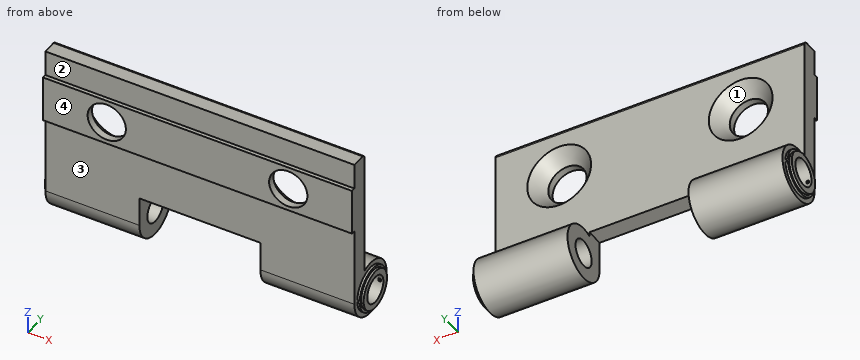
```python
from build123d import *

# Parameters (mm, degrees)
BOSS_EXTRUDE1_DEPTH    = 19.166666667
BOSS_EXTRUDE2_DEPTH    = 0.5
SKETCH3_W              = 5.123475383
SKETCH3_H              = 3.5
BOSS_EXTRUDE3_DEPTH    = 24.666666667
BOSS_EXTRUDE4_START    = 19.166666667
BOSS_EXTRUDE4_DEPTH    = 19.166666667
BOSS_EXTRUDE5_START    = 0.5
BOSS_EXTRUDE5_DEPTH    = 0.5
BOSS_EXTRUDE6_START    = 0.5
BOSS_EXTRUDE6_DEPTH    = 0.5
CUT_EXTRUDE1_DEPTH     = 19.166666667
SKETCH8_W              = 63
SKETCH8_H              = 3.5
BOSS_EXTRUDE7_DEPTH    = 0.338316441
SKETCH9_W              = 63
SKETCH9_H              = 5.461791824
BOSS_EXTRUDE8_DEPTH    = 0.8
CUT_EXTRUDE2_DEPTH     = 5.123475383
SKETCH11_W             = 63
SKETCH11_H             = 4.3
BOSS_EXTRUDE9_DEPTH    = 25.538208176
CUT_EXTRUDE3_DEPTH     = 0.338316441
SKETCH13_W             = 63
SKETCH13_H             = 0.8
CUT_EXTRUDE4_DEPTH     = 10.788208176
SKETCH14_W             = 24.666666666
SKETCH14_H             = 3.5
CUT_EXTRUDE5_DEPTH     = 0.538208176
BOSS_EXTRUDE10_START   = 0.5
SKETCH15_R             = 4
SKETCH15_R_2           = 2.75
BOSS_EXTRUDE10_DEPTH   = 0.5
SKETCH16_R             = 4
BOSS_EXTRUDE11_DEPTH   = 0.5
SKETCH17_W             = 5.25
SKETCH17_H             = 0.8
CUT_EXTRUDE6_DEPTH     = 72.95832127
F_10_CLEARANCE_HOLE1_D = 5.5
HOLE1_AT_2_COUNT       = 2
HOLE1_AT_2_PITCH       = 37
FILLET1_R              = 0.8
SCALE1_SCALE           = 0.3333


with BuildPart() as part:
    # Sketch1 → Boss-Extrude1 (new body)
    with BuildSketch(Plane(origin=(-12.333333333, 0, 0), x_dir=(0, 0, -1), z_dir=(1, 0, 0))):
        with BuildLine():
            Line((-5.123475383, 3.5), (-5.123475383, 0))
            Line((-5.123475383, 0), (0, 0))
            ThreePointArc((0, 0), (3.102418411, 10.041475531), (-5.123475383, 3.5))
        make_face()
    extrude(amount=-BOSS_EXTRUDE1_DEPTH)

    # Sketch2 → Boss-Extrude2 (add)
    with BuildSketch(Plane.ZY.offset(31.5)):
        with BuildLine():
            Line((-0.3, 9.989988864), (-0.3, 8.233587387))
            ThreePointArc((-0.3, 8.233587387), (0, 8.25), (0.3, 8.233587387))
            Line((0.3, 8.233587387), (0.3, 9.989988864))
            ThreePointArc((0.3, 9.989988864), (4.5, 5.5), (0.3, 1.010011136))
            Line((0.3, 1.010011136), (0.3, 2.766412613))
            ThreePointArc((0.3, 2.766412613), (0, 2.75), (-0.3, 2.766412613))
            Line((-0.3, 2.766412613), (-0.3, 1.010011136))
            ThreePointArc((-0.3, 1.010011136), (-4.5, 5.5), (-0.3, 9.989988864))
        make_face()
    extrude(amount=BOSS_EXTRUDE2_DEPTH)

    # Sketch3 → Boss-Extrude3 (add)
    with BuildSketch(Plane(origin=(-12.333333333, 0, 0), x_dir=(0, 0, -1), z_dir=(1, 0, 0))):
        with Locations((-2.561737692, 1.75)):
            Rectangle(SKETCH3_W, SKETCH3_H)
    extrude(amount=BOSS_EXTRUDE3_DEPTH)

    # Sketch4 → Boss-Extrude4 (add)
    with BuildSketch(Plane(origin=(12.333333333, 0, 0), x_dir=(0, 0, -1), z_dir=(1, 0, 0)).offset(BOSS_EXTRUDE4_START)):
        with BuildLine():
            Line((0, 0), (-5.123475383, 0))
            Line((-5.123475383, 0), (-5.123475383, 3.5))
            ThreePointArc((-5.123475383, 3.5), (3.102418411, 10.041475531), (0, 0))
        make_face()
        with BuildLine():
            Line((-1.887458609, 3.5), (0, 3.5))
            Line((0, 3.5), (0, 2.75))
            ThreePointArc((0, 2.75), (1.015504801, 8.055631038), (-1.887458609, 3.5))
        make_face(mode=Mode.SUBTRACT)
    extrude(amount=-BOSS_EXTRUDE4_DEPTH)

    # Sketch5 → Boss-Extrude5 (add)
    with BuildSketch(Plane(origin=(31.5, 0, 0), x_dir=(0, 0, -1), z_dir=(1, 0, 0)).offset(BOSS_EXTRUDE5_START)):
        with BuildLine():
            Line((-0.3, 9.989988864), (-0.3, 8.233587387))
            ThreePointArc((-0.3, 8.233587387), (-2.75, 5.5), (-0.3, 2.766412613))
            Line((-0.3, 2.766412613), (-0.3, 1.010011136))
            ThreePointArc((-0.3, 1.010011136), (-4.5, 5.5), (-0.3, 9.989988864))
        make_face()
    extrude(amount=-BOSS_EXTRUDE5_DEPTH)

    # Sketch6 → Boss-Extrude6 (add)
    with BuildSketch(Plane(origin=(31.5, 0, 0), x_dir=(0, 0, -1), z_dir=(1, 0, 0)).offset(BOSS_EXTRUDE6_START)):
        with BuildLine():
            Line((0.3, 1.010011136), (0.3, 2.766412613))
            ThreePointArc((0.3, 2.766412613), (2.75, 5.5), (0.3, 8.233587387))
            Line((0.3, 8.233587387), (0.3, 9.989988864))
            ThreePointArc((0.3, 9.989988864), (4.5, 5.5), (0.3, 1.010011136))
        make_face()
    extrude(amount=-BOSS_EXTRUDE6_DEPTH)

    # Sketch7 → Cut-Extrude1 (cut)
    with BuildSketch(Plane(origin=(31.5, 0, 0), x_dir=(0, 0, -1), z_dir=(1, 0, 0))):
        with BuildLine():
            Line((0, 3.5), (-1.887458609, 3.5))
            ThreePointArc((-1.887458609, 3.5), (-1.015504801, 2.944368962), (0, 2.75))
            Line((0, 2.75), (0, 3.5))
        make_face()
    extrude(amount=-CUT_EXTRUDE1_DEPTH, mode=Mode.SUBTRACT)

    # Sketch8 → Boss-Extrude7 (add)
    with BuildSketch(Plane.XY.offset(5.123475383)):
        with Locations((0, 1.75)):
            Rectangle(SKETCH8_W, SKETCH8_H)
    extrude(amount=BOSS_EXTRUDE7_DEPTH)

    # Sketch9 → Boss-Extrude8 (add)
    with BuildSketch(Plane.XZ):
        with Locations((0, 2.730895912)):
            Rectangle(SKETCH9_W, SKETCH9_H)
    extrude(amount=BOSS_EXTRUDE8_DEPTH)

    # Sketch10 → Cut-Extrude2 (cut)
    with BuildSketch(Plane(origin=(0, 0, 0), x_dir=(-1, 0, 0), z_dir=(0, 0, -1))):
        Polygon((12.333333333, 3.5), (-12.333333333, 3.5), (-12.333333333, 0), (-31.5, 0), (-31.5, -0.8), (31.5, -0.8), (31.5, 0), (12.333333333, 0), align=None)
    extrude(amount=-CUT_EXTRUDE2_DEPTH, mode=Mode.SUBTRACT)

    # Sketch11 → Boss-Extrude9 (add)
    with BuildSketch(Plane.XY.offset(5.461791824)):
        with Locations((0, 1.35)):
            Rectangle(SKETCH11_W, SKETCH11_H)
    extrude(amount=BOSS_EXTRUDE9_DEPTH)

    # Sketch12 → Cut-Extrude3 (cut)
    with BuildSketch(Plane(origin=(0, 0, 5.123475383), x_dir=(-1, 0, 0), z_dir=(0, 0, -1))):
        Polygon((12.333333333, 3.5), (-12.333333333, 3.5), (-12.333333333, 0), (-31.5, 0), (-31.5, -0.8), (31.5, -0.8), (31.5, 0), (12.333333333, 0), align=None)
    extrude(amount=-CUT_EXTRUDE3_DEPTH, mode=Mode.SUBTRACT)

    # Sketch13 → Cut-Extrude4 (cut)
    with BuildSketch(Plane(origin=(0, 0, 5.461791824), x_dir=(-1, 0, 0), z_dir=(0, 0, -1))):
        with Locations((0, -0.4)):
            Rectangle(SKETCH13_W, SKETCH13_H)
    extrude(amount=-CUT_EXTRUDE4_DEPTH, mode=Mode.SUBTRACT)

    # Sketch14 → Cut-Extrude5 (cut)
    with BuildSketch(Plane(origin=(0, 0, 5.461791824), x_dir=(-1, 0, 0), z_dir=(0, 0, -1))):
        with Locations((0, 1.75)):
            Rectangle(SKETCH14_W, SKETCH14_H)
    extrude(amount=-CUT_EXTRUDE5_DEPTH, mode=Mode.SUBTRACT)

    # Sketch15 → Boss-Extrude10 (add)
    with BuildSketch(Plane(origin=(32, 0, 0), x_dir=(0, 0, -1), z_dir=(1, 0, 0)).offset(BOSS_EXTRUDE10_START)):
        with Locations(Location((0, 5.5, 0), (0, 0, 94.301222305))):
            Circle(SKETCH15_R)
        with Locations((0, 5.5)):
            Circle(SKETCH15_R_2, mode=Mode.SUBTRACT)
    extrude(amount=-BOSS_EXTRUDE10_DEPTH)

    # Sketch16 → Boss-Extrude11 (add)
    with BuildSketch(Plane.ZY.offset(32)):
        with Locations(Location((0, 5.5, 0), (0, 0, 85.698777695))):
            Circle(SKETCH16_R)
    extrude(amount=BOSS_EXTRUDE11_DEPTH)

    # Sketch17 → Cut-Extrude6 (cut, through all)
    with BuildSketch(Plane(origin=(31.5, 0, 0), x_dir=(0, 0, -1), z_dir=(1, 0, 0))):
        with Locations((-28.375, -0.4)):
            Rectangle(SKETCH17_W, SKETCH17_H)
    extrude(amount=-CUT_EXTRUDE6_DEPTH, mode=Mode.SUBTRACT)

    # #10 Clearance Hole1 (through all)
    with Locations(Plane.ZY.offset(32.5)):
        with Locations((0, 5.5)):
            Hole(F_10_CLEARANCE_HOLE1_D / 2)

    # Sketch20 → Hole1 (revolve, cut)
    with BuildSketch(Plane(origin=(18.5, 3.5, 21), x_dir=(0, 0, 1), z_dir=(1, 0, 0))):
        Polygon((0, 0), (0, 4.3), (3.9, 4.3), (3.9, 2.8), (6.5, 0), align=None)
    hole1 = revolve(axis=Axis((18.5, 9.945314094, 21), (0, -1, 0)), mode=Mode.SUBTRACT)

    # Hole1 at 2: Hole1 ×2
    with Locations(*[(-i * HOLE1_AT_2_PITCH, 0, 0) for i in range(1, HOLE1_AT_2_COUNT)]):
        add(hole1, mode=Mode.SUBTRACT)

    # Fillet1
    fillet1_edges = [part.edges().sort_by_distance(p)[0] for p in [
        (0, 3.5, 31),
    ]]
    fillet(fillet1_edges, radius=FILLET1_R)


with BuildPart() as part_1:
    # Scale1: scaled about (0, 2.846153953, 11.820192401)
    add(part.part.scale(SCALE1_SCALE).moved(Location((0, 1.89753084, 7.880522274))))


solid = part_1.part
```
Verification items for the finished model (mm, model axes). Face numbers are marked on the shaded views. A direction names the side the tool comes from. Coordinates: 2 decimals unless noted, no trailing zeros. Write each loop counter-clockwise with the first axis right and the second up, starting at its lowest first coordinate (ties: lowest second). Pieces come first, ordered by that corner, then holes. Notation, with made-up numbers: (71.25, 33.5) - (123.25, 33.5) arc R28 cw to (123.25, 66.5) - close; hole circle Ø6 at (21, 26.5). An arc over 180 degrees is marked (long way). Write item = value, one per line.
Q1. Cross-section at A-A (y = 4.85). Give the number of separate pieces and of enclosed holes in the cut face, plus the area to 3 significant figures.
Answer:
separate_pieces = 2
enclosed_holes = 2
area = 38.2 mm²
Q2. Cross-section at C-C (x = -2.5). Enter the section's corners in (y, z), plus the area to 3 significant figures.
Answer:
outline = (1.63, 13.3) - (1.9, 13.3) - (1.9, 9.88) - (3.06, 9.88) - (3.06, 17.95) arc R0.27 ccw to (2.8, 18.21) - (1.9, 18.21) - (1.9, 16.46) - (1.63, 16.46) - close
area = 10.5 mm²
Q3. Mould release check, pull along Z, two halves, no side actions. Record for the marked faces 1 and 2: released by +Z, released by -Z, zero draft, split by the parting line, or undercut.
Answer:
face_1 = undercut
face_2 = zero draft
Q4. Access from +Z, -Z, +X, -X, +Y, -Y to the whole of each face (thin tool, end or side, straight path). Record for the marked faces 3 and 4.
Answer:
face_3 = -Z, +X, -X, -Y
face_4 = +Z, -Z, +X, -X, -Y
Q5. Material ranges on L1, parallel to Z at x = -6.25, y = 3.75; L2, parallel to Z at x = 5, y = 2.9; L3, parallel to X at y = 2.2, z = 8.25, recorded low to high. Write a range as from..to.
Answer:
L1 = 6.05..6.96, 8.8..9.71
L2 = 6.25..7.49, 8.27..13.24, 16.52..18.19
L3 = -10.5..-4.11, 4.11..10.5
